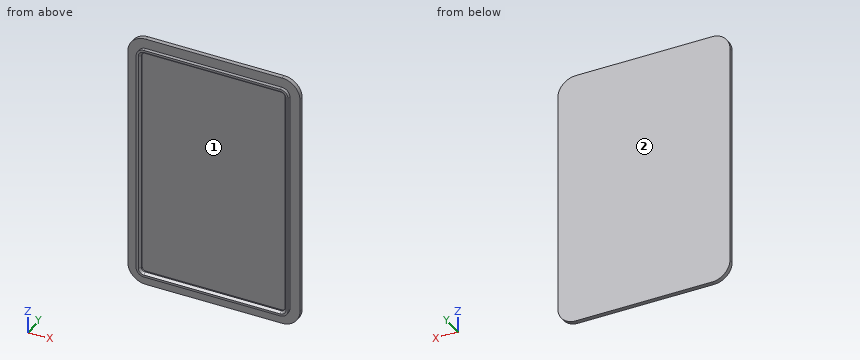
Autodesk Inventor part; units mm, degrees
ref_plane "YZ Plane" through (0, 0, 0) normal (1, 0, 0) x (0, 1, 0)
ref_plane "XZ Plane" through (0, 0, 0) normal (0, 1, 0) x (-1, 0, 0)
ref_plane "XY Plane" through (0, 0, 0) normal (0, 0, 1) x (1, 0, 0)
sketch "Sketch1" plane through (0, 0, 0) normal (0, 1, 0) x (-1, 0, 0)
  line L0 (4.7625, 0) -> (53.0225, 0)
  line L1 (57.785, -4.7625) -> (57.785, -85.4075)
  line L2 (53.0225, -90.17) -> (4.7625, -90.17)
  line L3 (0, -85.4075) -> (0, -4.7625)
  arc A0 (57.785, -4.7625) -> (53.0225, 0) centre (53.0225, -4.7625) ccw
  arc A1 (4.7625, 0) -> (0, -4.7625) centre (4.7625, -4.7625) ccw
  arc A2 (0, -85.4075) -> (4.7625, -90.17) centre (4.7625, -85.4075) ccw
  arc A3 (53.0225, -90.17) -> (57.785, -85.4075) centre (53.0225, -85.4075) ccw
  line L4 (56.1975, -85.4075) -> (56.1975, -4.7625)
  arc A4 (56.1975, -4.7625) -> (53.0225, -1.5875) centre (53.0225, -4.7625) ccw
  line L5 (53.0225, -1.5875) -> (4.7625, -1.5875)
  arc A5 (4.7625, -1.5875) -> (1.5875, -4.7625) centre (4.7625, -4.7625) ccw
  line L6 (1.5875, -4.7625) -> (1.5875, -85.4075)
  arc A6 (1.5875, -85.4075) -> (4.7625, -88.5825) centre (4.7625, -85.4075) ccw
  line L7 (4.7625, -88.5825) -> (53.0225, -88.5825)
  arc A7 (53.0225, -88.5825) -> (56.1975, -85.4075) centre (53.0225, -85.4075) ccw
  line L8 (59.3725, -85.4075) -> (59.3725, -4.7625)
  arc A8 (59.3725, -4.7625) -> (53.0225, 1.5875) centre (53.0225, -4.7625) ccw
  line L9 (53.0225, 1.5875) -> (4.7625, 1.5875)
  arc A9 (4.7625, 1.5875) -> (-1.5875, -4.7625) centre (4.7625, -4.7625) ccw
  line L10 (-1.5875, -4.7625) -> (-1.5875, -85.4075)
  arc A10 (-1.5875, -85.4075) -> (4.7625, -91.7575) centre (4.7625, -85.4075) ccw
  line L11 (4.7625, -91.7575) -> (53.0225, -91.7575)
  arc A11 (53.0225, -91.7575) -> (59.3725, -85.4075) centre (53.0225, -85.4075) ccw
  line L12 (54.2925, -4.7625) -> (54.2925, -85.4075)
  arc A12 (53.0225, -86.6775) -> (54.2925, -85.4075) centre (53.0225, -85.4075) ccw
  line L13 (53.0225, -86.6775) -> (4.7625, -86.6775)
  arc A13 (3.4925, -85.4075) -> (4.7625, -86.6775) centre (4.7625, -85.4075) ccw
  line L14 (3.4925, -85.4075) -> (3.4925, -4.7625)
  arc A14 (4.7625, -3.4925) -> (3.4925, -4.7625) centre (4.7625, -4.7625) ccw
  line L15 (4.7625, -3.4925) -> (53.0225, -3.4925)
  arc A15 (54.2925, -4.7625) -> (53.0225, -3.4925) centre (53.0225, -4.7625) ccw
  line L16 (55.8165, -4.7625) -> (55.8165, -85.4075)
  arc A16 (53.0225, -88.2015) -> (55.8165, -85.4075) centre (53.0225, -85.4075) ccw
  line L17 (53.0225, -88.2015) -> (4.7625, -88.2015)
  arc A17 (1.9685, -85.4075) -> (4.7625, -88.2015) centre (4.7625, -85.4075) ccw
  line L18 (1.9685, -85.4075) -> (1.9685, -4.7625)
  arc A18 (4.7625, -1.9685) -> (1.9685, -4.7625) centre (4.7625, -4.7625) ccw
  line L19 (4.7625, -1.9685) -> (53.0225, -1.9685)
  arc A19 (55.8165, -4.7625) -> (53.0225, -1.9685) centre (53.0225, -4.7625) ccw
  point P0 (0, 0)
  point P1 (0, 0)
  point P2 (57.785, -90.17)
  point P3 (57.785, 0)
  point P4 (0, -90.17)
  dimension "d0" = 90.17
  dimension "d1" = 57.785
  dimension "d2" = 4.7625
  dimension "d3" = 1.5875
  dimension "d4" = 1.5875
  dimension "d5" = 1.905
  dimension "d6" = 0.381
extrude "Extrusion1" add sketch "Sketch1" along normal blind 1.524 contours L0 A0 L1 A3 L2 A2 L3 A1 | A7 L7 A6 L6 A5 L5 A4 L4 | A11 L11 A10 L10 A9 L9 A8 L8 | L12 A12 L13 A13 L14 A14 L15 A15 | L16 A16 L17 A17 L18 A18 L19 A19
extrude "Extrusion2" add sketch "Sketch1" against normal blind 1.27 contours L16 A16 L17 A17 L18 A18 L19 A19
chamfer "Chamfer1" distance 0.762 angle 45 8 edges at (-28.8925, -1.27, -3.4925) (-3.8645, -1.27, -3.8645) (-3.4925, -1.27, -45.085) (-3.8645, -1.27, -86.3055) (-28.8925, -1.27, -86.6775) (-53.9205, -1.27, -86.3055) (-54.2925, -1.27, -45.085) (-53.9205, -1.27, -3.8645)
equation "\"d3\" = d4"
properties part number "BatteryCaseSide3"
For this review, take the finished solid that the model builds, in its own axes (mm). Face numbers are marked on the shaded views. Give positions to 0.01 mm unless a question says otherwise; leave off trailing zeros. Write each loop counter-clockwise with the first axis right and the second up, starting at its lowest first coordinate (ties: lowest second). Pieces come first, ordered by that corner, then holes. Notation, with made-up numbers: M 6,18.5 L 49,18.5 A18 cw 49,43.5 Z; hole C 32,45.5 d8. An arc over 180 degrees is marked long. Answer as a JSON object with one key per item and string values. Group by question number.
Item 1: Draft analysis for pull direction X (two halves, no side actions). For the marked faces 1 and 2, state which applies: +X half, -X half, draft (parallel to the pull), parting line (faces both ways), or undercut.
Item 2: For probe 1 along Z at (x, y) = (-23.5, -0.3); probe 2 along X at (y, z) = (-0.1, -65.5); probe 3 along Y at (x, z) = (-44, -78), list the stretches that pass through material, from the lowest coordinate up. Write a range as [from, to].
Item 3: Consider section A-A on z = -40. Write out the cut boundary in (x, y).
Item 4: Consider section B-B on x = -25. Write out the cut boundary in (y, z), plus the area to 3 significant figures.
Item 5: For pin 1 Ø0.6 at (y, z) = (-1, -41) entering from +X; pin 2 Ø12 at (x, z) = (-12, -10.5) entering from -Y; pin 3 Ø0.6 at (x, y) = (-22.5, -0.5) entering from -Z, all flat-tipped, find the tip position at first contact; note any pin that passes through.
Check result:
{
 "1": {"face 1": "undercut", "face 2": "draft"},
 "2": {"probe 1": "z = [-88.2, -86.68], [-3.49, -1.97]", "probe 2": "x = [-55.82, -54.29], [-3.49, -1.97]", "probe 3": "y = [0, 1.52]"},
 "3": {"outline": "M -59.37,0 L -55.82,0 L -55.82,-1.27 L -55.05,-1.27 L -54.29,-0.51 L -54.29,0 L -3.49,0 L -3.49,-0.51 L -2.73,-1.27 L -1.97,-1.27 L -1.97,0 L 1.59,0 L 1.59,1.52 L -59.37,1.52 Z"},
 "4": {"outline": "M -1.27,-88.2 L 0,-88.2 L 0,-91.76 L 1.52,-91.76 L 1.52,1.59 L 0,1.59 L 0,-1.97 L -1.27,-1.97 L -1.27,-2.73 L -0.51,-3.49 L 0,-3.49 L 0,-86.68 L -0.51,-86.68 L -1.27,-87.44 Z", "area": "146 mm^2"},
 "5": {"pin 1": "stops at x = -1.97", "pin 2": "stops at y = 0", "pin 3": "stops at z = -88.2"}
}
